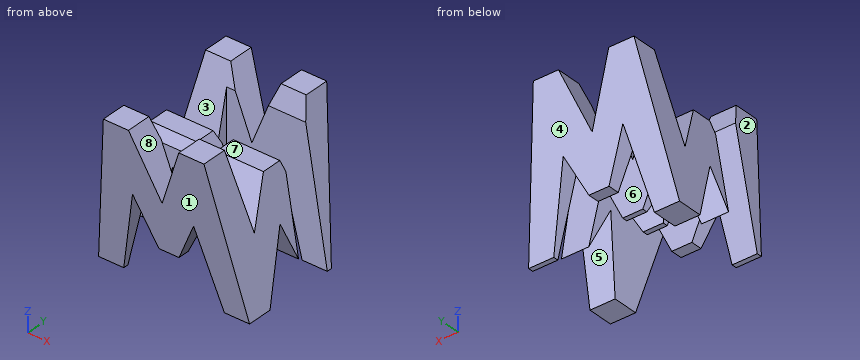
```python
from build123d import *

# Parameters (mm, degrees)
F0_W      = 38.1
F0_H      = 38.1
F1_DEPTH  = 38.1
F6_DEPTH  = 76.2
F8_DEPTH  = 38.1
F9_W      = 25.4
F9_H      = 7.62
F10_DEPTH = 38.1


with BuildPart() as f1:
    # F0 (on Front) → F1 (new body)
    with BuildSketch(Plane.XZ):
        with Locations((-19.05, 19.05)):
            Rectangle(F0_W, F0_H)
    extrude(amount=F1_DEPTH)

    # F5 (on offset) → F6 (cut)
    with BuildSketch(Plane.YZ.offset(38.1)):
        Polygon((-11.43, 16.465984), (-6.35, 38.1), (-31.75, 38.1), (-26.67, 17.490659), (-21.59, 28.575), (-16.51, 28.575), align=None)
        Polygon((-25.4, 0), (-12.7, 0), (-19.05, 15.875), align=None)
        Polygon((-6.35, 0), (0, 0), (0, 38.1), align=None)
        Polygon((-38.1, 0), (-31.75, 0), (-38.1, 38.1), align=None)
    extrude(amount=-F6_DEPTH, mode=Mode.SUBTRACT)

    # F7 (on offset) → F8 (cut)
    with BuildSketch(Plane.XZ.offset(38.1)):
        Polygon((-38.1, 38.1), (-38.1, 0), (-31.75, 38.1), align=None)
        Polygon((-19.05, 22.225), (-12.7, 38.1), (-25.4, 38.1), align=None)
        Polygon((-6.35, 38.1), (0, 0), (0, 38.1), align=None)
        Polygon((-31.75, 0), (-6.35, 0), (-11.43, 19.911673), (-16.51, 9.525), (-21.59, 9.525), (-26.67, 21.155922), align=None)
    extrude(amount=-F8_DEPTH, mode=Mode.SUBTRACT)

    # F9 (on offset) → F10 (cut)
    with BuildSketch(Plane.XY.offset(38.1)):
        with Locations((-12.7, -11.43)):
            Rectangle(F9_W, F9_H)
        with Locations((-25.4, -26.67)):
            Rectangle(F9_W, F9_H)
    extrude(amount=-F10_DEPTH, mode=Mode.SUBTRACT)


solid = f1.part
```
Check sheet for the modelled part. Datum: model origin and axes. Units: mm. Face numbers are marked on the shaded views. A direction names the side the tool comes from. Round coordinates to 2 decimals unless told otherwise and drop trailing zeros. Loops run counter-clockwise (first coordinate to the right, second up) from the corner with the lowest first, then second, coordinate; pieces in that order, holes last. Notation, with made-up numbers: (-30.5, -9.75) - (-9.5, -9.75) arc R34 cw to (-9.5, 24.25) - close; hole circle Ø1 at (59.25, 48). An arc over 180 degrees is marked (long way). Answer as a JSON object with one key per item and string values. Group by question number.
Q1. Sectioned sample at B-B, the plane x = -14. Count the separate pieces of the cut face and the enclosed holes in it, plus the area to 3 significant figures.
Q2. Gauge pin test, flat ends, axial feed: P1, Ø4, axis at x = -8.5, y = -18, coming from the +Z side (3 decimals); P2, Ø1, axis at x = -18, y = -16, coming from the -Z side (3 decimals); P3, Ø1, axis at x = -31, z = 13.5, coming from the -Y side. Record the tip position at first contact, or that the pin passes through.
Q3. Set-up check for the marked faces 5, 6, 7 and 8: record each of +Z, -Z, +X, -X, +Y, -Y from which the full face is reachable in a straight line by a thin tool's end or side.
Q4. Sectioned sample at C-C, the plane y = -7. Enter the section's corners in (x, z) (3 decimals).
Q5. Sectioned sample at A-A, the plane z = 34. Enter the section's corners in (x, y).
Q6. Sectioned sample at D-D, the plane x = -26. Enter the section's corners in (y, z) (3 decimals), plus the area to 3 significant figures.
Q7. Mould release check, pull along Y, two halves, no side actions. Record for the marked faces 1, 2, 3 and 4: released by +Y, released by -Y, zero draft, split by the parting line, or undercut.
Q8. Scan lines: line 1 along Y through (x, z) = (-12.5, 20); line 2 along Y through (x, z) = (-3.5, 18); line 3 along X through (y, z) = (-33, 10). Record each from-to range of solid material in increasing order. Write a range as [from, to].
Solution:
{
 "1": {"separate pieces": "3", "enclosed holes": "0", "area": "319 mm²"},
 "2": {"P1": "stops at z = 28.575", "P2": "stops at z = 9.525", "P3": "stops at y = -34.08"},
 "3": {"face 5": "-Z, +X, -X", "face 6": "+Z, -Z, +X", "face 7": "+Z, +X, -X", "face 8": "+Z, +Y, -Y"},
 "4": {"outline": "(-38.1, 0) - (-31.75, 0) - (-26.67, 21.156) - (-21.59, 9.525) - (-16.51, 9.525) - (-11.43, 19.912) - (-6.35, 0) - (0, 0) - (-5.889, 35.332) - (-13.807, 35.332) - (-19.05, 22.225) - (-24.293, 35.332) - (-32.211, 35.332) - close"},
 "5": {"outline": "(-32.43, -37.42) - (-23.76, -37.42) - (-23.76, -30.74) - (-32.43, -30.74) - close; (-32.43, -7.31) - (-23.76, -7.31) - (-23.76, -0.68) - (-32.43, -0.68) - close; (-14.34, -37.42) - (-5.67, -37.42) - (-5.67, -30.74) - (-14.34, -30.74) - close; (-14.34, -7.31) - (-5.67, -7.31) - (-5.67, -0.68) - (-14.34, -0.68) - close"},
 "6": {"outline": "(-38.1, 38.1) - (-35.02, 19.622) - (-30.48, 19.622) - (-30.48, 32.948) - (-31.75, 38.1) - close; (-22.86, 19.622) - (-12.754, 19.622) - (-16.51, 28.575) - (-21.59, 28.575) - (-22.86, 25.804) - close; (-10.689, 19.622) - (-3.08, 19.622) - (0, 38.1) - (-6.35, 38.1) - close", "area": "310 mm²"},
 "7": {"face 1": "released by -Y", "face 2": "zero draft", "face 3": "undercut", "face 4": "released by +Y"},
 "8": {"line 1": "y = [-35.08, -27.29], [-25.52, -15.24], [-7.62, -3.02]", "line 2": "y = [-34.75, -26.8], [-26.44, -15.24], [-7.62, -3.35]", "line 3": "x = [-36.43, -29.35], [-21.8, -16.28], [-8.9, -1.67]"}
}
